Print and shaded views of the part. All mm, measured from the part's lowest x, y and z. A direction names the side the tool comes from. Round coordinates to 2 decimals unless told otherwise and drop trailing zeros. Loops run counter-clockwise (first coordinate to the right, second up) from the corner with the lowest first, then second, coordinate; pieces in that order, holes last. Notation, with made-up numbers: (33, 35.25) -> (72, 35.25) arc R34 cw to (72, 67.25) -> close; hole circle Ø6 at (27.5, 65.5). An arc over 180 degrees is marked (long way). Use a Markdown table: item, result.
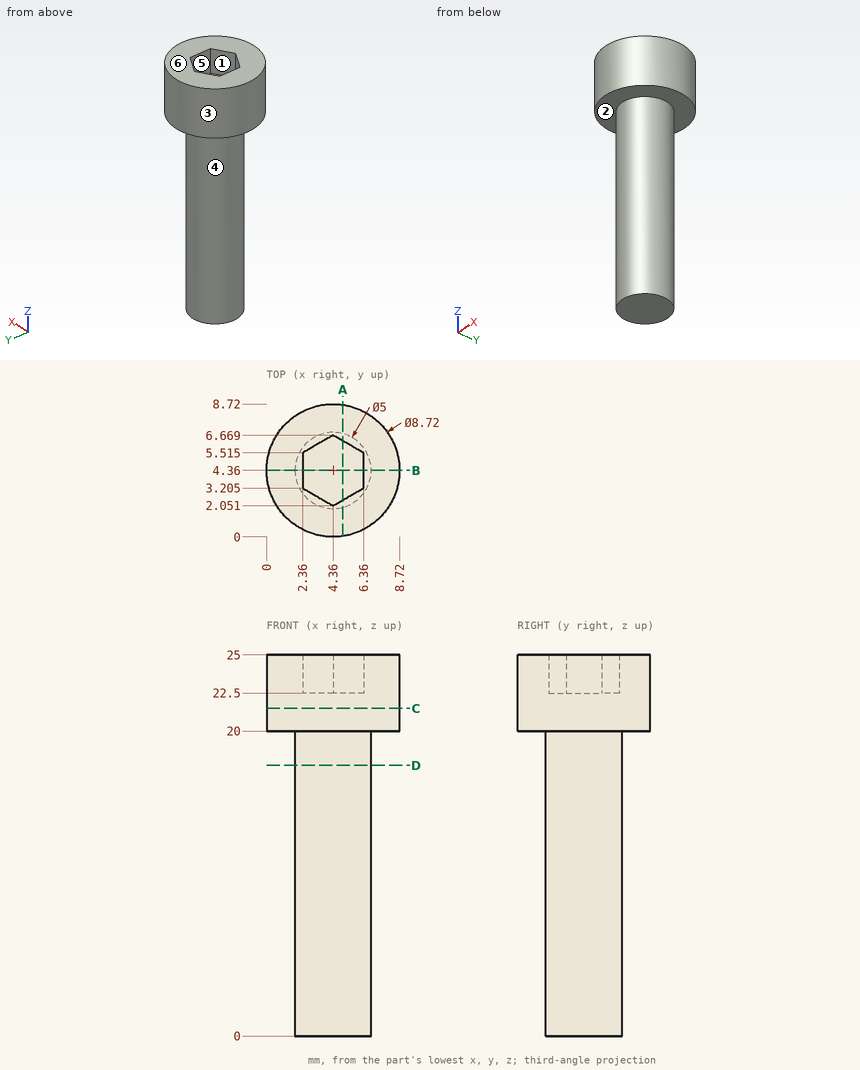
Q1. Band-saw the part on B-B, the plane y = 4.36. Give the cut face in (x, z), plus the area to 3 significant figures.
Results list:
| item | result |
|---|---|
| outline | (0, 20) -> (1.86, 20) -> (1.86, 0) -> (6.86, 0) -> (6.86, 20) -> (8.72, 20) -> (8.72, 25) -> (6.36, 25) -> (6.36, 22.5) -> (2.36, 22.5) -> (2.36, 25) -> (0, 25) -> close |
| area | 134 mm² |
Q2. Flat gauge pins, fed straight in: pin 1 (2 mm diameter, centred on x = 6, z = 10.5, fed in from +Y); pin 2 (1.5 mm diameter, centred on y = 2.5, z = 19, fed in from -X); pin 3 (1.5 mm diameter, centred on x = 2.5, z = 20.5, fed in from -Y). Where does each tip first touch, or does it go through?
Results list:
| item | result |
|---|---|
| pin 1 | stops at y = 6.78 |
| pin 2 | stops at x = 2.12 |
| pin 3 | stops at y = 0.14 |
Q3. Band-saw the part on C-C, the plane z = 21.5. Give the cut face in (x, y).
Results list:
| item | result |
|---|---|
| outline | circle Ø8.72 at (4.36, 4.36) |
Q4. Tool access for the marked faces 1, 2 and 3: list every direction of +Z, -Z, +X, -X, +Y, -Y with a clear straight run to the whole face (end or side of a thin tool).
Results list:
| item | result |
|---|---|
| face 1 | +Z |
| face 2 | -Z |
| face 3 | +Z, -Z |
Q5. Drill centre lines: L1, parallel to Z at x = 6.5, y = 0.75; L2, parallel to Z at x = 3, y = 4; L3, parallel to Y at x = 6, z = 21.5. Where is each one in solid material? Low to high. Write a range as from..to.
Results list:
| item | result |
|---|---|
| L1 | z = 20..25 |
| L2 | z = 0..22.5 |
| L3 | y = 0.32..8.4 |
Q6. Band-saw the part on D-D, the plane z = 17.75. Give the cut face in (x, y).
Results list:
| item | result |
|---|---|
| outline | circle Ø5 at (4.36, 4.36) |
Q7. Pull direction X, two halves, no side cores. Call the marked faces 4, 5 and 6: released by +X, released by -X, zero draft, split by the parting line, or undercut.
Results list:
| item | result |
|---|---|
| face 4 | split by the parting line |
| face 5 | undercut |
| face 6 | zero draft |
Q8. Band-saw the part on A-A, the plane x = 5. Give the cut face in (y, z).
Results list:
| item | result |
|---|---|
| outline | (0.05, 20) -> (1.94, 20) -> (1.94, 0) -> (6.78, 0) -> (6.78, 20) -> (8.67, 20) -> (8.67, 25) -> (6.3, 25) -> (6.3, 22.5) -> (2.42, 22.5) -> (2.42, 25) -> (0.05, 25) -> close |
